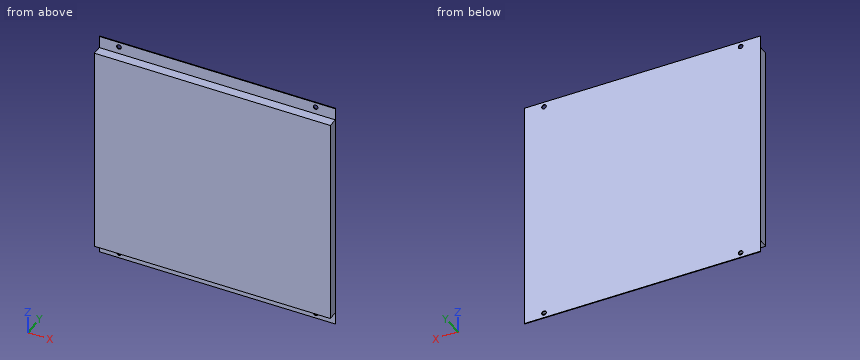
from build123d import *

# Parameters (mm, degrees)
BOX001_W      = 460
BOX001_H      = 18.5
BOX001_DEPTH  = 24
BOX_W         = 460
BOX_H         = 18.5
BOX_DEPTH     = 24
SKETCH_W      = 457.2
SKETCH_H      = 457.2
SKETCH_R      = 4.5
EXTRUDE_DEPTH = 20


with BuildPart() as cube001:
    # Box001 → Box001 (new body)
    with BuildSketch(Plane(origin=(-229, 0, 205), x_dir=(1, 0, 0), z_dir=(0, 0, 1))):
        with Locations((230, 9.25)):
            Rectangle(BOX001_W, BOX001_H)
    extrude(amount=BOX001_DEPTH)


with BuildPart() as cut:
    # Box → Box (new body)
    with BuildSketch(Plane(origin=(-229, 0, -229), x_dir=(1, 0, 0), z_dir=(0, 0, 1))):
        with Locations((230, 9.25)):
            Rectangle(BOX_W, BOX_H)
    extrude(amount=BOX_DEPTH)

    # Fusion: union Cube001
    add(cube001.part)


with BuildPart() as cut_body:
    # Sketch → Extrude (new body)
    with BuildSketch(Plane.XZ):
        Rectangle(SKETCH_W, SKETCH_H)
        with Locations((-190.5, -219.075)):
            Circle(SKETCH_R, mode=Mode.SUBTRACT)
        with Locations((-190.5, 219.075)):
            Circle(SKETCH_R, mode=Mode.SUBTRACT)
        with Locations((190.5, 219.075)):
            Circle(SKETCH_R, mode=Mode.SUBTRACT)
        with Locations((190.5, -219.075)):
            Circle(SKETCH_R, mode=Mode.SUBTRACT)
    extrude(amount=-EXTRUDE_DEPTH)

    # Cut: cut cut
    add(cut.part, mode=Mode.SUBTRACT)


solid = cut_body.part
Geometry: final body of the model. Coordinates: model frame, mm. Round coordinates to 2 decimals unless told otherwise and drop trailing zeros. Order: outer loops, then holes, each group sorted by start corner. A loop starts at its lowest first (then second) coordinate and runs counter-clockwise, first axis right, second up.
Q1. Section B-B, the plane y = 5.25. Output: boundary loops of the cut face in (x, z), and give its area (3 significant figures).
Result sheet:
outline: (-228.6, -205) - (228.6, -205) - (228.6, 205) - (-228.6, 205) - close
area: 187,000 mm2
Q2. Section A-A, the plane x = 31.5. Output: boundary loops of the cut face in (y, z).
Result sheet:
outline: (0, -205) - (18.5, -205) - (18.5, -228.6) - (20, -228.6) - (20, 228.6) - (18.5, 228.6) - (18.5, 205) - (0, 205) - close
Q3. Pin query (flat end, axial travel): pin 1 (5 mm diameter, centred on x = -71.5, y = 10.5, fed in from +Z); pin 2 (12 mm diameter, centred on x = 75, z = 214, fed in from -Y); pin 3 (8 mm diameter, centred on x = -190.5, z = 219.075, fed in from -Y); pin 4 (10 mm diameter, centred on x = -21, z = -179, fed in from -Y). Return the tip coordinate at first contact, or that it passes through.
Result sheet:
pin 1: stops at z = 205
pin 2: stops at y = 18.5
pin 3: passes through
pin 4: stops at y = 0
Q4. Material intervals for probe 1 along Z at (x, y) = (-190.5, 19.1) (3 decimals); probe 2 along Z at (x, y) = (166.5, 11.75), sorted ascending.
Result sheet:
probe 1: z = -228.6 to -223.575, -214.575 to 214.575, 223.575 to 228.6
probe 2: z = -205 to 205
